```python
from build123d import *

# Parameters (mm, degrees)
F1_DEPTH      = 2.286
F2_W          = 1.27
F2_H          = 17.78
F3_DEPTH      = 6.35
F3_DEPTH_BACK = 2.286
F4_D          = 1.6933333333


# Not quite as in the source:
# - a feature names something its author has since deleted; it is built from what else it names


with BuildPart() as f1:
    # F0 (on Top) → F1 (new body)
    with BuildSketch(Plane.XY):
        Polygon((-39.7502322496, -19.8751161248), (-31.0001806734, -29.1251689516), (73.3058652154, -29.1251689516), (101.3186621261, 20.063493978), (101.3186621261, 25.3395497125), (78.8771229202, 34.0285638846), (72.3271246897, 39.6729167182), (52.3297434038, 47.023841916), (50.4247434038, 47.023841916), (21.8864718038, 47.023841916), (19.9814718038, 47.023841916), (-8.5567997962, 47.023841916), (-12.4402794499, 23.3751358177), (-17.5001015898, 6.8750406358), (-33.2501941145, 0), (-48.0002794499, -4.3750257881), align=None)
    extrude(amount=F1_DEPTH)

    # F2 (on face) → F3 (join, two sides)
    with BuildSketch(Plane.XY.offset(2.286)) as f3_sk:
        with Locations((79.6558652154, 6.4348310484)):
            Rectangle(F2_W, F2_H)
        Polygon((-32.2015322451, -27.8551689516), (-31.0001806734, -29.1251689516), (73.3058652154, -29.1251689516), (74.0291264296, -27.8551689516), align=None)
        Polygon((80.2908652154, 30.5648310484), (-11.2596214034, 30.5648310484), (-11.4681748498, 29.2948310484), (79.0208652154, 29.2948310484), (79.0208652154, 27.7073310484), (80.2908652154, 27.7073310484), align=None)
        Polygon((-34.0091347846, -0.2251095453), (-34.0091347846, -25.944275189), (-32.7391347846, -27.2868463713), (-32.7391347846, 0.2230814616), (-33.2501941145, 0), align=None)
    extrude(amount=F3_DEPTH)
    extrude(f3_sk.sketch, amount=-F3_DEPTH_BACK)

    # F4 (through all)
    with Locations(Plane.XY.offset(2.286)):
        with Locations((-41.6291347846, -13.7730257881), (-41.6291347846, -8.6930257881), (-41.6291347846, -3.6130257881), (-3.5502565962, 43.2212361431), (-3.5502565962, 38.1412361431), (-3.5502565962, 33.0612361431), (24.3897434038, 43.2212361431), (24.3897434038, 38.1412361431), (24.3897434038, 33.0612361431), (52.3297434038, 42.9037361431), (52.3297434038, 37.8237361431), (52.3297434038, 32.7437361431), (86.6408652154, 23.6032530031), (86.6408652154, 18.5232530031), (86.6408652154, 13.4432530031)):
            Hole(F4_D / 2)


solid = f1.part
```
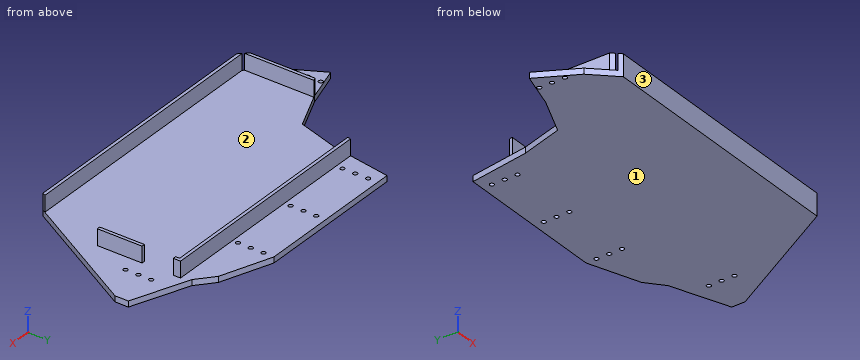
Can you work these out from the model? Positions are in its coordinate system, mm. Face numbers are marked on the shaded views. Coordinates: 2 decimals unless noted, no trailing zeros. Loops run counter-clockwise (first coordinate to the right, second up) from the corner with the lowest first, then second, coordinate; pieces in that order, holes last.
1) For pin 1 (1 mm diameter, centred on x = 50, z = 3, fed in from +Y); pin 2 (2 mm diameter, centred on y = 7, z = 2.5, fed in from -X); pin 3 (12 mm diameter, centred on x = 40, y = -12, fed in from -Z); pin 4 (1 mm diameter, centred on x = 80, z = 6, fed in from -Y), each with a flat end and sliding along its axis, tell me the tip position at first contact or that it passes through.
2) Imagine slicing it at A-A on z = 5.5. List the corners of the cut face in (x, y) for me.
3) Imagine slicing it at B-B on x = 11. List the corners of the cut face in (y, z) for me, plus the area to 3 significant figures.
4) Imagine slicing it at C-C on x = 60. List the corners of the cut face in (y, z) for me.
5) I need wall thicknesses on probe 1 along Y at (x, z) = (67, 4.75); probe 2 along X at (y, z) = (-17.5, 6.5); probe 3 along Z at (x, y) = (20, 13.5). Which ranges of each line are inside material? Lowest first, please.
6) Thinking about a two-plate mould opening in Y: for the marked faces 1, 2 and 3, which applies, pulls with the +Y half, pulls with the -Y half, needs draft (parallel to the pull), parting line crosses it, or undercut?
7) Imagine slicing it at D-D on x = -37.5. List the corners of the cut face in (y, z) for me.
Completed:
1. pin 1: stops at y = 30.56
1. pin 2: stops at x = -19.45
1. pin 3: stops at z = 0
1. pin 4: stops at y = -2.46
2. outline: (-34.01, -25.94) - (-32.74, -27.29) - (-32.74, 0.22) - (-33.25, 0) - (-34.01, -0.23) - close; (-32.2, -27.86) - (-31, -29.13) - (73.31, -29.13) - (74.03, -27.86) - close; (-11.47, 29.29) - (79.02, 29.29) - (79.02, 27.71) - (80.29, 27.71) - (80.29, 30.56) - (-11.26, 30.56) - close; (79.02, -2.46) - (80.29, -2.46) - (80.29, 15.32) - (79.02, 15.32) - close
3. outline: (-29.13, 0) - (47.02, 0) - (47.02, 2.29) - (30.56, 2.29) - (30.56, 8.64) - (29.29, 8.64) - (29.29, 2.29) - (-27.86, 2.29) - (-27.86, 8.64) - (-29.13, 8.64) - close
3. area: 190 mm2
4. outline: (-29.13, 0) - (44.2, 0) - (44.2, 2.29) - (30.56, 2.29) - (30.56, 8.64) - (29.29, 8.64) - (29.29, 2.29) - (-27.86, 2.29) - (-27.86, 8.64) - (-29.13, 8.64) - close
5. probe 1: y = -29.13 to -27.86, 29.29 to 30.56
5. probe 2: x = -34.01 to -32.74
5. probe 3: z = 0 to 2.29
6. face 1: needs draft
6. face 2: undercut
6. face 3: pulls with the -Y half
7. outline: (-22.25, 0) - (-1.26, 0) - (-1.26, 2.29) - (-22.25, 2.29) - close
